```python
from build123d import *

# Parameters (mm, degrees)
F2_R     = 22
F3_DEPTH = 25
F4_SIZE  = 1


with BuildPart() as f1:
    # F0 (on Front) → F1 (revolve)
    with BuildSketch(Plane.XZ):
        Polygon((0, 14), (0, 0), (25.75, 0), (27.75, 2.5), (29.75, 2.5), (29.75, 4), (27.75, 4), (27.75, 14), align=None)
    revolve(axis=Axis((0, 0, 7), (0, 0, -1)))

    # F2 (on face) → F3 (cut)
    with BuildSketch(Plane.XY.offset(14)):
        Circle(F2_R)
    extrude(amount=-F3_DEPTH, mode=Mode.SUBTRACT)

    # F4
    f4_edges = [f1.edges().sort_by_distance(p)[0] for p in [
        (-27.75, 0, 14),
    ]]
    chamfer(f4_edges, length=F4_SIZE)


solid = f1.part
```
CAD build for the part. Positions are in the model's coordinates, mm. A direction names the side the tool comes from. Round coordinates to 2 decimals unless told otherwise and drop trailing zeros. Order: outer loops, then holes, each group sorted by start corner. A loop starts at its lowest first (then second) coordinate and runs counter-clockwise, first axis right, second up.
Q1. Wall check: L1, parallel to Y at x = 0, z = 8.5; L2, parallel to Z at x = -20, y = 21; L3, parallel to Y at x = -7, z = 9. Give the ranges that are in metal, low to high.
Q2. Two-plate mould, pull along Y, no slides. Class faces 1 (the flat face through (-20, 20, 2.5)), 2 (the cylindrical face through (-4.769, -21.477, 7.098)), 3 (the cylindrical face through (26.469, -8.335, 8.563)): pulls with the +Y half, pulls with the -Y half, needs draft (parallel to the pull), parting line crosses it, or undercut.
Q3. Drop flat-ended pins along their axis: pin 1 (1.5 mm diameter, centred on y = 0, z = 11, fed in from +X); pin 2 (1.5 mm diameter, centred on y = 2, z = 7, fed in from -X); pin 3 (8 mm diameter, centred on y = 23, z = 5, fed in from +X). Give the stop position or say it passes through.
Q4. Slice it at A-A (x = 0). Write the cut outline in (y, z).
Q5. Slice it at C-C (z = 11.25). Write the cut outline in (x, y), and give its area (3 significant figures).
Q6. Which spindle directions (+Z, -Z, +X, -X, +Y, -Y) get a long thin tool onto all of the face, cutting with end or side? Do faces 4 (the flat face through (20, 20, 4)), 5 (the conical face through (-5.6, 25.3, 0.2)). Say none if no direction does.
Results below:
1. L1: y = -27.75 to -22, 22 to 27.75
1. L2: z = 2.5 to 4
1. L3: y = -26.85 to -20.86, 20.86 to 26.85
2. face 1: needs draft
2. face 2: undercut
2. face 3: parting line crosses it
3. pin 1: stops at x = 27.75
3. pin 2: stops at x = -27.72
3. pin 3: stops at x = 22.79
4. outline: (-29.75, 2.5) - (-27.75, 2.5) - (-25.75, 0) - (-22, 0) - (-22, 14) - (-26.75, 14) - (-27.75, 13) - (-27.75, 4) - (-29.75, 4) - close; (22, 0) - (25.75, 0) - (27.75, 2.5) - (29.75, 2.5) - (29.75, 4) - (27.75, 4) - (27.75, 13) - (26.75, 14) - (22, 14) - close
5. outline: circle Ø55.5 at (0, 0); hole circle Ø44 at (0, 0)
5. area: 899 mm2
6. face 4: +Z
6. face 5: -Z
